from build123d import *

# Parameters (mm, degrees)
F0_W     = 12.822116
F0_H     = 31.884328
F1_DEPTH = 38.1
F2_W     = 12.712212
F2_H     = 31.884328
F3_DEPTH = 6.35
F4_W     = 12.712212
F4_H     = 31.884328
F5_DEPTH = 6.35


with BuildPart() as f1:
    # F0 (on Right) → F1 (new body)
    with BuildSketch(Plane.YZ):
        with Locations((32.140768, 15.942164)):
            Rectangle(F0_W, F0_H)
    extrude(amount=F1_DEPTH)

    # F2 (on face) → F3 (join)
    with BuildSketch(Plane(origin=(0, 38.551826, 0), x_dir=(-1, 0, 0), z_dir=(0, 1, 0))):
        with Locations((-31.743894, 15.942164)):
            Rectangle(F2_W, F2_H)
    extrude(amount=F3_DEPTH)

    # F4 (on face) → F5 (join)
    with BuildSketch(Plane.XZ.offset(-25.72971)):
        with Locations((31.743894, 15.942164)):
            Rectangle(F4_W, F4_H)
    extrude(amount=F5_DEPTH)


solid = f1.part
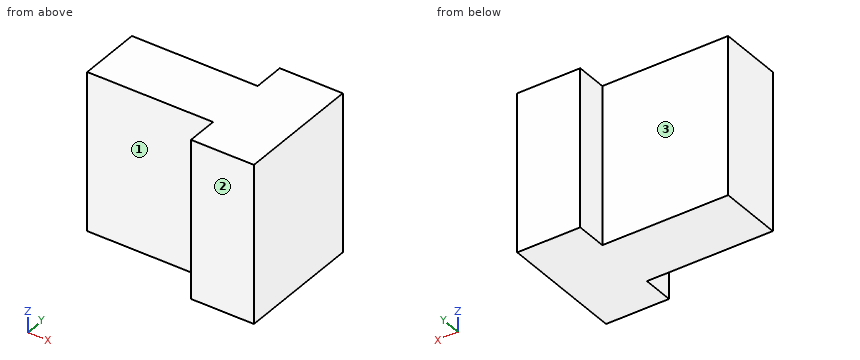
Check sheet for the modelled part. Datum: model origin and axes. Units: mm. Face numbers are marked on the shaded views. A direction names the side the tool comes from. Round coordinates to 2 decimals unless told otherwise and drop trailing zeros. Order: outer loops, then holes, each group sorted by start corner. A loop starts at its lowest first (then second) coordinate and runs counter-clockwise, first axis right, second up.
(1) Cross-section at C-C, the plane x = 11.5. Enter the section's corners in (y, z), and give its area (3 significant figures).
(2) Go/stop test with flat-tipped pins: P1, Ø12.5, axis at x = 11.5, z = 9, coming from the -Y side; P2, Ø12.5, axis at x = 11.5, z = 19, coming from the +Y side; P3, Ø1.9, axis at y = 21.5, z = 9.5, coming from the -X side. Record where each tip stops, or that it passes through.
(3) Cross-section at A-A, the plane z = 24.5. Enter the section's corners in (x, y).
(4) Access from +Z, -Z, +X, -X, +Y, -Y to the whole of each face (thin tool, end or side, straight path). Record for the marked faces 1, 2 and 3.
(5) Scan lines: probe 1 along X at (y, z) = (39, 12); probe 2 along Y at (x, z) = (23, 13). Record each from-to range of solid material in increasing order.
(6) Cross-section at B-B, the plane y = 39.75. Enter the section's corners in (x, z).
Check sheet entries:
1. outline: (25.73, 0) - (38.55, 0) - (38.55, 31.88) - (25.73, 31.88) - close
1. area: 409 mm2
2. P1: stops at y = 25.73
2. P2: stops at y = 38.55
2. P3: stops at x = 25.39
3. outline: (0, 25.73) - (25.39, 25.73) - (25.39, 19.38) - (38.1, 19.38) - (38.1, 44.9) - (25.39, 44.9) - (25.39, 38.55) - (0, 38.55) - close
4. face 1: +Z, -Z, -X, -Y
4. face 2: +Z, -Z, +X, -X, -Y
4. face 3: +Z, -Z, -X, +Y
5. probe 1: x = 25.39 to 38.1
5. probe 2: y = 25.73 to 38.55
6. outline: (25.39, 0) - (38.1, 0) - (38.1, 31.88) - (25.39, 31.88) - close
